Read the model definition and answer for the solid it produces. Units are mm, in the model's axes. Give positions to 0.01 mm unless a question says otherwise; leave off trailing zeros. Order: outer loops, then holes, each group sorted by start corner. A loop starts at its lowest first (then second) coordinate and runs counter-clockwise, first axis right, second up. Notation, with made-up numbers: (72, 67) - (91, 67) arc R25 ccw to (91, 100) - close; hole circle Ø7 at (2.5, 76.5). An arc over 180 degrees is marked (long way). One line per item, written item: value. Start each with the question number.
```python
from build123d import *

# Parameters (mm, degrees)
EXTRUDE_2_DEPTH     = 60
SKETCH_3_R          = 3
CUT_EXTRUDE_1_DEPTH = 3.5
SKETCH_4_R          = 1.75
CUT_EXTRUDE_2_DEPTH = 3
FILLET_1_R          = 1


with BuildPart() as part:
    # 草图2 → 凸台-拉伸2 (new body)
    with BuildSketch(Plane.XY):
        Polygon((0, 0), (9, 0), (9, 3.5), (8.646446609, 3.853553391), (8.146446609, 3.853553391), (8.146446609, 4.353553391), (8.646446609, 4.353553391), (9, 4.707106781), (9, 6.5), (0, 6.5), (0, 4.707106781), (0.353553391, 4.353553391), (0.853553391, 4.353553391), (0.853553391, 3.853553391), (0.353553391, 3.853553391), (0, 3.5), align=None)
    extrude(amount=-EXTRUDE_2_DEPTH)

    # 草图3 → 切除-拉伸1 (cut)
    with BuildSketch(Plane(origin=(0, 6.5, 0), x_dir=(1, 0, 0), z_dir=(0, 1, 0))):
        with Locations(Location((4.5, 5, 0), (0, 0, 270))):
            Circle(SKETCH_3_R)
        with Locations(Location((4.5, 25, 0), (0, 0, 270))):
            Circle(SKETCH_3_R)
        with Locations(Location((4.5, 45, 0), (0, 0, 270))):
            Circle(SKETCH_3_R)
        with Locations((4.5, 65)):
            Circle(SKETCH_3_R)
        with Locations((4.5, 85)):
            Circle(SKETCH_3_R)
        with Locations((4.5, 105)):
            Circle(SKETCH_3_R)
        with Locations((4.5, 125)):
            Circle(SKETCH_3_R)
        with Locations((4.5, 145)):
            Circle(SKETCH_3_R)
        with Locations((4.5, 165)):
            Circle(SKETCH_3_R)
        with Locations((4.5, 185)):
            Circle(SKETCH_3_R)
        with Locations((4.5, 205)):
            Circle(SKETCH_3_R)
        with Locations((4.5, 225)):
            Circle(SKETCH_3_R)
    extrude(amount=-CUT_EXTRUDE_1_DEPTH, mode=Mode.SUBTRACT)

    # 草图4 → 切除-拉伸2 (cut)
    with BuildSketch(Plane(origin=(0, 3, 0), x_dir=(1, 0, 0), z_dir=(0, 1, 0))):
        with Locations(Location((4.5, 5, 0), (0, 0, 270))):
            Circle(SKETCH_4_R)
        with Locations(Location((4.5, 25, 0), (0, 0, 270))):
            Circle(SKETCH_4_R)
        with Locations(Location((4.5, 45, 0), (0, 0, 270))):
            Circle(SKETCH_4_R)
        with Locations((4.5, 65)):
            Circle(SKETCH_4_R)
        with Locations((4.5, 85)):
            Circle(SKETCH_4_R)
        with Locations((4.5, 105)):
            Circle(SKETCH_4_R)
        with Locations((4.5, 125)):
            Circle(SKETCH_4_R)
        with Locations((4.5, 145)):
            Circle(SKETCH_4_R)
        with Locations((4.5, 165)):
            Circle(SKETCH_4_R)
        with Locations((4.5, 185)):
            Circle(SKETCH_4_R)
        with Locations((4.5, 205)):
            Circle(SKETCH_4_R)
        with Locations((4.5, 225)):
            Circle(SKETCH_4_R)
    extrude(amount=-CUT_EXTRUDE_2_DEPTH, mode=Mode.SUBTRACT)

    # 圆角1
    fillet_1_edges = [part.edges().sort_by_distance(p)[0] for p in [
        (9, 1.75, -60),
        (0, 1.75, -60),
        (9, 1.75, 0),
        (0, 1.75, 0),
    ]]
    fillet(fillet_1_edges, radius=FILLET_1_R)


solid = part.part
```
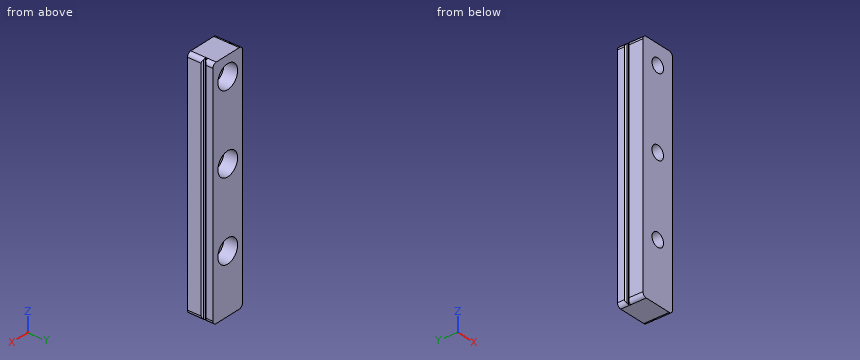
1) Each of these flat-tipped pins is pushed along its axis until it touches: pin 1 (0.6 mm diameter, centred on y = 4, z = -39, fed in from +X); pin 2 (3 mm diameter, centred on x = 4.5, z = -46, fed in from +Y). Where does it stop, or does it pass through?
2) Section C-C on y = 1.5 is taken. Write down the section's boundary in (x, z).
3) Section B-B on z = -45 is taken. Write down the section's boundary in (x, y), plus the area to 3 significant figures.
4) Section A-A on x = 4.5 is taken. Write down the section's boundary in (y, z).
5) Find the intervals of material crossed by probe 1 along Z at (x, y) = (4.75, 6); probe 2 along X at (y, z) = (4.9, -45); probe 3 along X at (y, z) = (1.4, -25), in increasing order. Write a range as from..to.
6) Section D-D on z = -29.5 is taken. Write down the section's boundary in (x, y).
Solved:
1. pin 1: stops at x = 8.8
1. pin 2: stops at y = 3
2. outline: (0, -59) arc R1 ccw to (1, -60) - (8, -60) arc R1 ccw to (9, -59) - (9, -1) arc R1 ccw to (8, 0) - (1, 0) arc R1 ccw to (0, -1) - close; hole circle Ø3.5 at (4.5, -45); hole circle Ø3.5 at (4.5, -25); hole circle Ø3.5 at (4.5, -5)
3. outline: (0, 0) - (2.75, 0) - (2.75, 3) - (1.5, 3) - (1.5, 6.5) - (0, 6.5) - (0, 4.71) - (0.35, 4.35) - (0.85, 4.35) - (0.85, 3.85) - (0.35, 3.85) - (0, 3.5) - close; (6.25, 0) - (9, 0) - (9, 3.5) - (8.65, 3.85) - (8.15, 3.85) - (8.15, 4.35) - (8.65, 4.35) - (9, 4.71) - (9, 6.5) - (7.5, 6.5) - (7.5, 3) - (6.25, 3) - close
3. area: 25.9 mm2
4. outline: (0, -60) - (6.5, -60) - (6.5, -48) - (3, -48) - (3, -46.75) - (0, -46.75) - close; (0, -43.25) - (3, -43.25) - (3, -42) - (6.5, -42) - (6.5, -28) - (3, -28) - (3, -26.75) - (0, -26.75) - close; (0, -23.25) - (3, -23.25) - (3, -22) - (6.5, -22) - (6.5, -8) - (3, -8) - (3, -6.75) - (0, -6.75) - close; (0, -3.25) - (3, -3.25) - (3, -2) - (6.5, -2) - (6.5, 0) - (0, 0) - close
5. probe 1: z = -60..-47.99, -42.01..-27.99, -22.01..-7.99, -2.01..0
5. probe 2: x = 0..1.5, 7.5..9
5. probe 3: x = 0..2.75, 6.25..9
6. outline: (0, 0) - (9, 0) - (9, 3.5) - (8.65, 3.85) - (8.15, 3.85) - (8.15, 4.35) - (8.65, 4.35) - (9, 4.71) - (9, 6.5) - (0, 6.5) - (0, 4.71) - (0.35, 4.35) - (0.85, 4.35) - (0.85, 3.85) - (0.35, 3.85) - (0, 3.5) - close
